Geometry: final body of the model. Coordinates: model frame, mm. Face numbers are marked on the shaded views. A direction names the side the tool comes from. Round coordinates to 2 decimals unless told otherwise and drop trailing zeros. Write each loop counter-clockwise with the first axis right and the second up, starting at its lowest first coordinate (ties: lowest second). Pieces come first, ordered by that corner, then holes. Notation, with made-up numbers: M 1,63.25 L 16,63.25 A19 cw 16,76.25 Z; hole C -20,-1.5 d6. An arc over 180 degrees is marked long. Put each result on its own line as item: value. Start each with the question number.
```python
from build123d import *

# Parameters (mm, degrees)
SKETCH1_W           = 6.35
SKETCH1_H           = 1.044000004
BOSS_EXTRUDE1_DEPTH = 6.35
EXTRUDE_THIN1_DEPTH = 6.096


with BuildPart() as part:
    # Sketch1 → Boss-Extrude1 (new body, symmetric)
    with BuildSketch(Plane(origin=(0, 0, 0), x_dir=(0, 0, -1), z_dir=(1, 0, 0))):
        with Locations((0, 0.522000002)):
            Rectangle(SKETCH1_W, SKETCH1_H)
    extrude(amount=BOSS_EXTRUDE1_DEPTH, both=True)

    # Sketch2 → Extrude-Thin1 (add, symmetric)
    with BuildSketch(Plane(origin=(0, 0, 0), x_dir=(0, 0, -1), z_dir=(1, 0, 0))):
        Polygon((3.175, 0.522000002), (4.064, 0.522000002), (4.064, 0), (4.953, 0), (4.953, 0.127), (4.191, 0.127), (4.191, 0.649000002), (3.175, 0.649000002), align=None)
    extrude_thin1 = extrude(amount=EXTRUDE_THIN1_DEPTH, both=True)

    # Mirror1: Extrude-Thin1 across plane
    add(extrude_thin1.mirror(Plane.XY))


solid = part.part
```
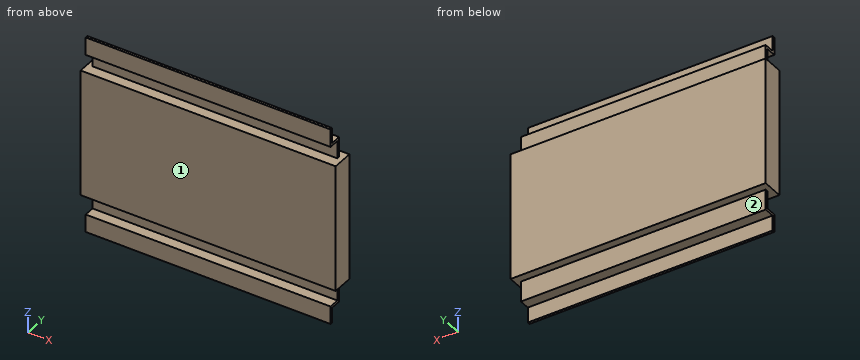
1) First-contact query: pin 1 (0.6 mm diameter, centred on x = 1.5, y = 0.5, fed in from +Z); pin 2 (0.5 mm diameter, centred on x = -2.5, z = -3.5, fed in from +Y); pin 3 (0.5 mm diameter, centred on y = 0, z = -4, fed in from +X). Flat tips, straight axial feed; report the tip coordinate or a pass-through.
2) Ray query, probe 1 along Z at (x, y) = (-3.75, 0.95) (3 decimals); probe 2 along X at (y, z) = (0.6, -3.25); probe 3 along Z at (x, y) = (-5.75, 0.6). Return the intervals inside material, ascending.
3) Access query for the marked faces 1 and 2. Directions: +Z, -Z, +X, -X, +Y, -Y. A direction counts if a zero-diameter tool reaches every point of the face in a straight line with its end or side. Return the directions, or none.
4) Section A-A, the plane y = 0.35. Output: boundary loops of the cut face in (x, z) (3 decimals), and give its area (3 significant figures).
5) Section C-C, the plane z = -3.5. Output: boundary loops of the cut face in (x, y).
6) Section B-B, the plane x = 0. Output: boundary loops of the cut face in (y, z) (3 decimals).
Solved:
1. pin 1: stops at z = 4.19
1. pin 2: stops at y = 0.65
1. pin 3: stops at x = 6.1
2. probe 1: z = -3.175 to 3.175
2. probe 2: x = -6.1 to 6.1
2. probe 3: z = -4.19 to 4.19
3. face 1: +Z, -Z, +X, -X, -Y
3. face 2: -Z, +X, -X, +Y
4. outline: M -6.35,-3.175 L 6.35,-3.175 L 6.35,3.175 L -6.35,3.175 Z; M -6.096,-4.191 L 6.096,-4.191 L 6.096,-4.064 L -6.096,-4.064 Z; M -6.096,4.064 L 6.096,4.064 L 6.096,4.191 L -6.096,4.191 Z
4. area: 83.7 mm2
5. outline: M -6.1,0.52 L 6.1,0.52 L 6.1,0.65 L -6.1,0.65 Z
6. outline: M 0,-4.953 L 0.127,-4.953 L 0.127,-4.191 L 0.649,-4.191 L 0.649,-3.175 L 1.044,-3.175 L 1.044,3.175 L 0.649,3.175 L 0.649,4.191 L 0.127,4.191 L 0.127,4.953 L 0,4.953 L 0,4.064 L 0.522,4.064 L 0.522,3.175 L 0,3.175 L 0,-3.175 L 0.522,-3.175 L 0.522,-4.064 L 0,-4.064 Z
